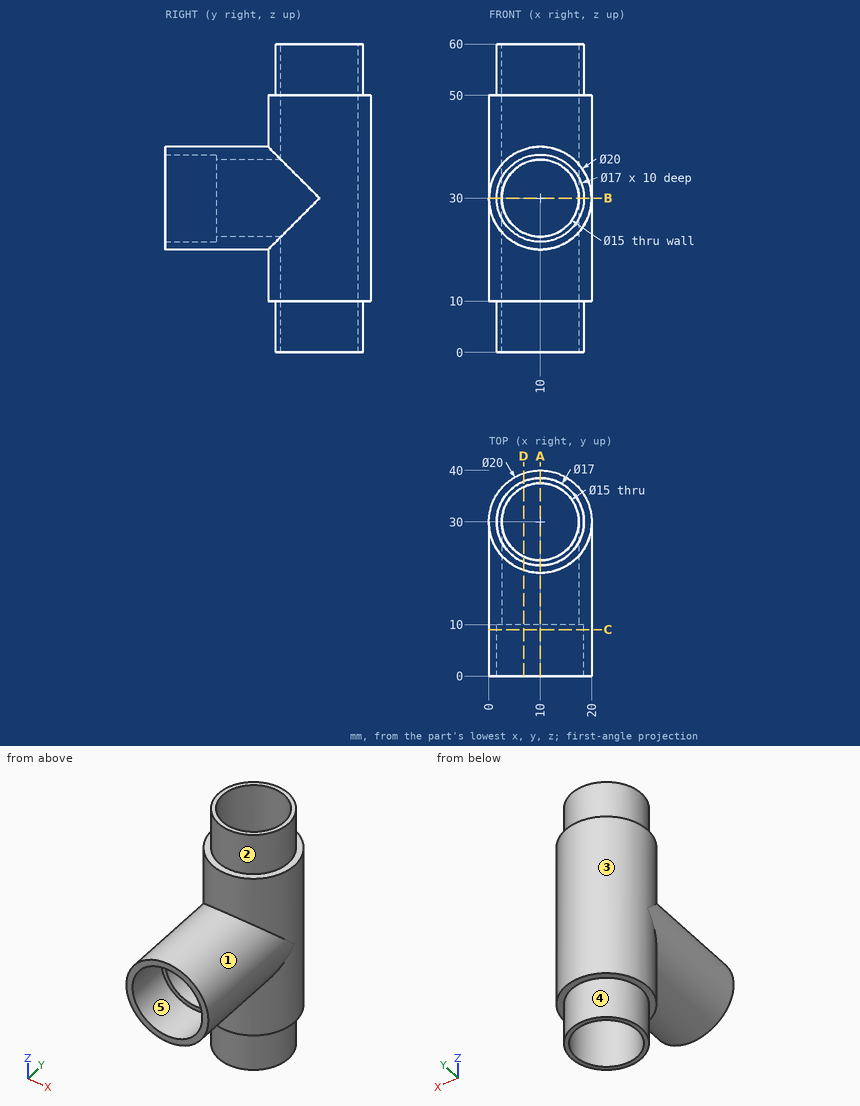
Answer from the drawing. Dimensions are ordinates in mm from the lowest x, y and z of the part. A direction names the side the tool comes from. Round coordinates to 2 decimals unless told otherwise and drop trailing zeros. Order: outer loops, then holes, each group sorted by start corner. A loop starts at its lowest first (then second) coordinate and runs counter-clockwise, first axis right, second up. Notation, with made-up numbers: (26, 69) - (74, 69) arc R26 cw to (74, 95) - close; hole circle Ø11 at (48, 31.25). An arc over 180 degrees is marked (long way). Put each result on its own line as item: value. Start each with the question number.
(1) For the marked faces 1, 2 and 3, determine the directions among +Z, -Z, +X, -X, +Y, -Y from which every point of the face is accessible in a straight line to the end or side of a thin tool.
(2) Find section D-D (x = 6.75). Give the vertices of the cut face in (y, z).
(3) Find section B-B (z = 30). Give the vertices of the cut face in (x, y).
(4) Determine the mould class of the marked faces 4 and 5 for opening direction X: released by +X, released by -X, zero draft, split by the parting line, or undercut.
(5) Given P1, Ø1.5, axis at x = 10, z = 13, coming from the -Y side; P2, Ø10, axis at y = 14, z = 50, coming from the +X side (3 decimals); P3, Ø6, axis at x = 16.5, z = 28.5, coming from the +Y side; P4, Ø12, axis at y = 5, z = 39, coming from the +X side, each flat-ended and moving along its own axis, determine where each tip first touches the part or whether it passes through.
(6) Find section A-A (x = 10). Give the vertices of the cut face in (y, z).
(7) Straight lines are drawn through the part: probe 1 along Z at (x, y) = (10, 17); probe 2 along X at (y, z) = (25, 30); probe 3 along Z at (x, y) = (10, 4.75). For each, find the intervals that lie inside material, in ascending order. Write a range as from..to.
(8) Find section C-C (y = 9). Give the vertices of the cut face in (x, z).
Reply:
1. face 1: -Y
1. face 2: +Z
1. face 3: none
2. outline: (0, 20.54) - (20.54, 20.54) - (20.54, 10) - (22.15, 10) - (22.15, 0) - (23.24, 0) - (23.24, 23.24) - (10, 23.24) - (10, 22.15) - (0, 22.15) - close; (0, 37.85) - (10, 37.85) - (10, 36.76) - (23.24, 36.76) - (23.24, 60) - (22.15, 60) - (22.15, 50) - (20.54, 50) - (20.54, 39.46) - (0, 39.46) - close; (36.76, 0) - (37.85, 0) - (37.85, 10) - (39.46, 10) - (39.46, 50) - (37.85, 50) - (37.85, 60) - (36.76, 60) - close
3. outline: (0, 0) - (1.5, 0) - (1.5, 10) - (2.5, 10) - (2.5, 30) arc R7.5 cw to (17.5, 30) - (17.5, 10) - (18.5, 10) - (18.5, 0) - (20, 0) - (20, 30) arc R10 ccw to (0, 30) - close
4. face 4: split by the parting line
4. face 5: undercut
5. P1: y = 20
5. P2: through
5. P3: y = 39.37
5. P4: x = 19.54
6. outline: (0, 20) - (20, 20) - (20, 10) - (21.5, 10) - (21.5, 0) - (22.5, 0) - (22.5, 22.5) - (10, 22.5) - (10, 21.5) - (0, 21.5) - close; (0, 38.5) - (10, 38.5) - (10, 37.5) - (22.5, 37.5) - (22.5, 60) - (21.5, 60) - (21.5, 50) - (20, 50) - (20, 40) - (0, 40) - close; (37.5, 0) - (38.5, 0) - (38.5, 10) - (40, 10) - (40, 50) - (38.5, 50) - (38.5, 60) - (37.5, 60) - close
7. probe 1: 20..22.5, 37.5..40
7. probe 2: 0..2.5, 17.5..20
7. probe 3: 20..21.5, 38.5..40
8. outline: circle Ø20 at (10, 30); hole circle Ø17 at (10, 30)
